Work out the finished part from the listing and answer in its coordinate system (mm). A direction names the side the tool comes from. Round coordinates to 2 decimals unless told otherwise and drop trailing zeros. Write each loop counter-clockwise with the first axis right and the second up, starting at its lowest first coordinate (ties: lowest second). Pieces come first, ordered by that corner, then holes. Notation, with made-up numbers: M 5,56 L 10,56 A21 ccw 10,92 Z; hole C 37,-4.5 d5. An arc over 180 degrees is marked long. Answer in a Markdown table with one row per item.
```python
from build123d import *

# Parameters (mm, degrees)
F1_DEPTH  = 20
F2_R      = 2.75
F3_DEPTH  = 80.8829045103
F5_R      = 5
F6_DEPTH  = 29.3829045103
F7_R      = 5
F8_DEPTH  = 3.5
F9_SIZE   = 4.99999
F11_REACH = 132.6751363952


# Not quite as in the source:
# - a fillet or chamfer is up to 0.001 mm smaller than in the source, because OpenCascade refuses the exact size


with BuildPart() as f1:
    # F0 (on Top) → F1 (new body)
    with BuildSketch(Plane.XY):
        Polygon((24.1481456572, 6.4704761276), (0, 0), (0, -7.5), (20, -7.5), (20, -47.5), (0, -47.5), (0, -55), (25, -55), (30, -50), (30, -2.3142860312), (99.1807730799, 16.2226462474), (96.5925826289, 25.8819045103), (28.9777747887, 7.7645713531), (25.0954891121, 22.2534587474), (20.2658599807, 20.9593635219), align=None)
    extrude(amount=F1_DEPTH)

    # F2 (on face) → F3 (cut, through all)
    with BuildSketch(Plane.XZ.offset(55)):
        with Locations((10, 10)):
            Circle(F2_R)
    extrude(amount=-F3_DEPTH, mode=Mode.SUBTRACT)

    # F5 (on offset) → F6 (cut, through all)
    with BuildSketch(Plane.XZ.offset(3.5)):
        with Locations((10, 10)):
            Circle(F5_R)
    extrude(amount=-F6_DEPTH, mode=Mode.SUBTRACT)

    # F7 (on face) → F8 (cut)
    with BuildSketch(Plane.XZ.offset(55)):
        with Locations((10, 10)):
            Circle(F7_R)
    extrude(amount=-F8_DEPTH, mode=Mode.SUBTRACT)

    # F9 (size 5 in the source; OpenCascade refuses exactly that, so slightly less here)
    f9_edges = [f1.edges().sort_by_distance(p)[0] for p in [
        (62.785179, 16.823238, 0),
        (62.785179, 16.823238, 20),
        (12.074073, 3.235238, 20),
        (12.074073, 3.235238, 0),
        (22.680675, 21.606411, 20),
        (22.680675, 21.606411, 0),
    ]]
    chamfer(f9_edges, length=F9_SIZE)

    f11_end = Plane(origin=(30, -26.1571430156, 10), x_dir=(0, 0, 1), z_dir=(1, 0, 0))
    # F10 (on face) → F11 (cut, up to a plane its end follows)
    with BuildSketch(Plane(origin=(96.5925826289, 25.8819045103, 0), x_dir=(-0.2588190451, 0.9659258263, 0), z_dir=(0.9659258263, 0.2588190451, 0))):
        Polygon((-3, 13.7573593129), (-6.2426406871, 17), (-15, 17), (-15, 3), (-6.2426406871, 3), (-3, 6.2426406871), align=None)
    f11_long = extrude(amount=-F11_REACH, mode=Mode.PRIVATE)
    add(split(f11_long, bisect_by=f11_end, keep=Keep.TOP, mode=Mode.PRIVATE), mode=Mode.SUBTRACT)


solid = f1.part
```
1. Given pin 1 (1 mm diameter, centred on y = -45.5, z = 7, fed in from +X); pin 2 (1 mm diameter, centred on x = 78, y = 16.5, fed in from +Z); pin 3 (6 mm diameter, centred on x = 10, z = 10, fed in from -Y); pin 4 (17.5 mm diameter, centred on x = 53.5, y = 5, fed in from -Z), each flat-ended and moving along its own axis, determine where each tip first touches the part or whether it passes through.
Calculated:
| item | result |
|---|---|
| pin 1 | stops at x = 30 |
| pin 2 | stops at z = 19.75 |
| pin 3 | stops at y = -51.5 |
| pin 4 | stops at z = 0 |
2. The part is cut by section A-A (z = 10). Count the separate pieces of the cut face and the enclosed holes in it, plus the area to 3 significant figures.
Calculated:
| item | result |
|---|---|
| separate pieces | 3 |
| enclosed holes | 0 |
| area | 1,100 mm² |
3. Determine the mould class of faces 4 (the flat face through (64.156, 12.43, 15.356)), 5 (the flat face through (63.26, 16.95, 9.93)), 6 (the flat face through (65, 9, 3)) for opening direction X: released by +X, released by -X, zero draft, split by the parting line, or undercut.
Calculated:
| item | result |
|---|---|
| face 4 | released by +X |
| face 5 | undercut |
| face 6 | zero draft |
4. The part is cut by section D-D (x = 45). Determine the outline of the cut face in (y, z).
Calculated:
| item | result |
|---|---|
| outline | M 1.7,0 L 6.88,0 L 12.06,5 L 12.06,15 L 6.88,20 L 1.7,20 L 1.7,17 L 5.59,17 L 8.95,13.76 L 8.95,6.24 L 5.59,3 L 1.7,3 Z |
5. The part is cut by section B-B (x = 16.5). Determine the outline of the cut face in (y, z).
Calculated:
| item | result |
|---|---|
| outline | M -55,0 L -47.5,0 L -47.5,20 L -55,20 Z; M -7.5,0 L -0.76,0 L 4.42,5 L 4.42,15 L -0.76,20 L -7.5,20 Z |
6. Consider line 1 along Z through (x, y) = (10, -50.15); line 2 along X through (y, z) = (-1.75, 10); line 3 along X through (y, z) = (-6, 3.75). Determine where each line is inside the solid, lowest interval first. Write a range as from..to.
Calculated:
| item | result |
|---|---|
| line 1 | z = 0..7.25, 12.75..20 |
| line 2 | x = 0..5, 15..30 |
| line 3 | x = 0..30 |
7. A tool of negligible diameter and unlimited length cuts with its end or side. For faces 1 (the flat face through (63.896, 14.569, 2.535)), 2 (the flat face through (20, -27, 10)), 3 (the cylindrical face through (14.77, -0.63, 11.5)), from which of +Z, -Z, +X, -X, +Y, -Y can it reach the whole face along a straight path? Write none if from no direction.
Calculated:
| item | result |
|---|---|
| face 1 | -Z, +Y |
| face 2 | +Z, -Z, -X |
| face 3 | +Y |
8. The part is cut by section C-C (y = -45.5). Determine the outline of the cut face in (x, z).
Calculated:
| item | result |
|---|---|
| outline | M 20,0 L 30,0 L 30,20 L 20,20 Z |
